from build123d import *

# Parameters (mm, degrees)
SKETCH1_W           = 350
SKETCH1_H           = 56.2
BOSS_EXTRUDE1_DEPTH = 10
SKETCH2_W           = 56.2
SKETCH2_H           = 56.2
CUT_EXTRUDE1_DEPTH  = 5
SKETCH3_W           = 10
SKETCH3_H           = 56.2
BOSS_EXTRUDE2_DEPTH = 10
SKETCH4_W           = 10
SKETCH4_H           = 56.2
BOSS_EXTRUDE3_DEPTH = 10
CUT_EXTRUDE2_DEPTH  = 56.2
SKETCH6_W           = 10
SKETCH6_H           = 56.2
BOSS_EXTRUDE4_DEPTH = 10
SKETCH7_W           = 10
SKETCH7_H           = 56.2
BOSS_EXTRUDE5_DEPTH = 10
CUT_EXTRUDE3_DEPTH  = 56.2
SKETCH9_W           = 30
SKETCH9_H           = 30
CUT_EXTRUDE4_DEPTH  = 5
SKETCH10_R          = 3
CUT_EXTRUDE5_DEPTH  = 5
SKETCH11_W          = 2.5
SKETCH11_H          = 15
CUT_EXTRUDE6_DEPTH  = 7
SKETCH12_W          = 2.5
SKETCH12_H          = 15
CUT_EXTRUDE7_DEPTH  = 7
SKETCH14_W          = 279.3
SKETCH14_H          = 56.2
CUT_EXTRUDE10_DEPTH = 10


with BuildPart() as part:
    # Sketch1 → Boss-Extrude1 (new body)
    with BuildSketch(Plane.XY):
        Rectangle(SKETCH1_W, SKETCH1_H)
    extrude(amount=BOSS_EXTRUDE1_DEPTH)

    # Sketch2 → Cut-Extrude1 (cut)
    with BuildSketch(Plane.XY.offset(10)):
        Rectangle(SKETCH2_W, SKETCH2_H)
    extrude(amount=-CUT_EXTRUDE1_DEPTH, mode=Mode.SUBTRACT)

    # Sketch3 → Boss-Extrude2 (add)
    with BuildSketch(Plane(origin=(175, 0, 0), x_dir=(0, 0, -1), z_dir=(1, 0, 0))):
        with Locations((-5, 0)):
            Rectangle(SKETCH3_W, SKETCH3_H)
    extrude(amount=BOSS_EXTRUDE2_DEPTH)

    # Sketch4 → Boss-Extrude3 (add)
    with BuildSketch(Plane.XY.offset(10)):
        with Locations((180, 0)):
            Rectangle(SKETCH4_W, SKETCH4_H)
    extrude(amount=BOSS_EXTRUDE3_DEPTH)

    # Sketch5 → Cut-Extrude2 (cut)
    with BuildSketch(Plane(origin=(0, 28.1, 0), x_dir=(1, 0, 0), z_dir=(0, 1, 0))):
        Polygon((175, -20), (185, -10), (185, -20), align=None)
    extrude(amount=-CUT_EXTRUDE2_DEPTH, mode=Mode.SUBTRACT)

    # Sketch6 → Boss-Extrude4 (add)
    with BuildSketch(Plane.ZY.offset(175)):
        with Locations((5, 0)):
            Rectangle(SKETCH6_W, SKETCH6_H)
    extrude(amount=BOSS_EXTRUDE4_DEPTH)

    # Sketch7 → Boss-Extrude5 (add)
    with BuildSketch(Plane.XY.offset(10)):
        with Locations((-180, 0)):
            Rectangle(SKETCH7_W, SKETCH7_H)
    extrude(amount=BOSS_EXTRUDE5_DEPTH)

    # Sketch8 → Cut-Extrude3 (cut)
    with BuildSketch(Plane(origin=(0, 28.1, 0), x_dir=(1, 0, 0), z_dir=(0, 1, 0))):
        Polygon((-175, -20), (-185, -10), (-185, -20), align=None)
    extrude(amount=-CUT_EXTRUDE3_DEPTH, mode=Mode.SUBTRACT)

    # Sketch9 → Cut-Extrude4 (cut)
    with BuildSketch(Plane.XY.offset(5)):
        Rectangle(SKETCH9_W, SKETCH9_H)
    extrude(amount=-CUT_EXTRUDE4_DEPTH, mode=Mode.SUBTRACT)

    # Sketch10 → Cut-Extrude5 (cut)
    with BuildSketch(Plane.XY.offset(5)):
        with Locations((21.55, 21.55)):
            Circle(SKETCH10_R)
        with Locations((-21.55, -21.55)):
            Circle(SKETCH10_R)
        with Locations((-21.55, 21.55)):
            Circle(SKETCH10_R)
        with Locations((21.55, -21.55)):
            Circle(SKETCH10_R)
    extrude(amount=-CUT_EXTRUDE5_DEPTH, mode=Mode.SUBTRACT)

    # Sketch11 → Cut-Extrude6 (cut)
    with BuildSketch(Plane(origin=(97.5, 0, 97.5), x_dir=(0.7071067811865478, 0, -0.7071067811865472), z_dir=(0.7071067811865472, 0, 0.7071067811865478))):
        with Locations((116.672618896, 0)):
            Rectangle(SKETCH11_W, SKETCH11_H)
    extrude(amount=-CUT_EXTRUDE6_DEPTH, mode=Mode.SUBTRACT)

    # Sketch12 → Cut-Extrude7 (cut)
    with BuildSketch(Plane(origin=(-97.5, 0, 97.5), x_dir=(0.7071067811865478, 0, 0.7071067811865472), z_dir=(-0.7071067811865472, 0, 0.7071067811865478))):
        with Locations((-116.672618896, 0)):
            Rectangle(SKETCH12_W, SKETCH12_H)
    extrude(amount=-CUT_EXTRUDE7_DEPTH, mode=Mode.SUBTRACT)

    # Sketch14 → Cut-Extrude10 (cut)
    with BuildSketch(Plane.XY.offset(10)):
        with Locations((45.35, 0)):
            Rectangle(SKETCH14_W, SKETCH14_H)
    extrude(amount=-CUT_EXTRUDE10_DEPTH, mode=Mode.SUBTRACT)


with BuildPart() as body_2:
    # of the pieces the cut leaves, the one that is kept (cut_extrude10_keep)
    add(part.part.solids().sort_by_distance((-185, -28.1, 0))[0])


solid = body_2.part
Input: part model. Units: mm. Frame: model coordinates. A direction names the side the tool comes from. Round coordinates to 2 decimals unless told otherwise and drop trailing zeros. Write each loop counter-clockwise with the first axis right and the second up, starting at its lowest first coordinate (ties: lowest second). Pieces come first, ordered by that corner, then holes.
1) Contact query for flat-ended pins moving along their axis: P1, Ø3, axis at y = -10.5, z = 13, coming from the +X side; P2, Ø1.5, axis at x = -127, y = -22, coming from the +Z side. Output: stop coordinate, or through.
2) Cut plane B-B (y = 11.5). Return the cut outline in (x, z).
3) Cut plane A-A (y = 3.5). Return the cut outline in (x, z), then the cut area to 3 significant figures.
4) Cut plane D-D (x = -139). Return the cut outline in (y, z).
5) Draft query along X for faces 1 (the flat face through (-178.444, -0.105, 11.676)), 2 (the flat face through (-140, 28.1, 5)), 3 (the flat face through (-178, -7.5, 13)), 4 (the flat face through (-94.3, 0, 5)). Return one class per face: pulls with the +X half, pulls with the -X half, needs draft (parallel to the pull), parting line crosses it, or undercut.
6) Ray query, L1, parallel to Z at x = -108, y = -9; L2, parallel to X at y = 18, z = 12.5; L3, parallel to X at y = -14, z = 17.5. Return the intervals inside material, ascending.
7) Cut plane C-C (z = 18). Return the cut outline in (x, y).
8) Reachability of faces 5 (the flat face through (-134, 0, 10)), 6 (the flat face through (-139, 0, 0)), 7 (the flat face through (-178, 7.5, 13)) from +Z, -Z, +X, -X, +Y, -Y: full face, straight path, thin tool, end or side. Return the list, or none.
Geometry says:
1. P1: stops at x = -175
1. P2: stops at z = 10
2. outline: (-185, 0) - (-94.3, 0) - (-94.3, 10) - (-175, 10) - (-175, 20) - (-185, 10) - close
3. outline: (-185, 0) - (-94.3, 0) - (-94.3, 10) - (-175, 10) - (-175, 10.1) - (-175.93, 9.17) - (-180.88, 14.12) - (-185, 10) - close; (-179.12, 15.88) - (-175, 11.77) - (-175, 20) - close
3. area: 940 mm2
4. outline: (-28.1, 0) - (28.1, 0) - (28.1, 10) - (-28.1, 10) - close
5. face 1: undercut
5. face 2: needs draft
5. face 3: undercut
5. face 4: pulls with the +X half
6. L1: z = 0 to 10
6. L2: x = -182.5 to -175
6. L3: x = -177.5 to -175
7. outline: (-177, -28.1) - (-175, -28.1) - (-175, 28.1) - (-177, 28.1) - close
8. face 5: +Z, +X, +Y, -Y
8. face 6: -Z, +X, -X, +Y, -Y
8. face 7: none
